Input: part model. Units: mm. Frame: model coordinates. Face numbers are marked on the shaded views. A direction names the side the tool comes from. Coordinates: 2 decimals unless noted, no trailing zeros. One line per question, with ' | ' between items. Start each with the question number.
```python
from build123d import *

# Parameters (mm, degrees)
F0_W     = 60
F0_H     = 52.3357634497
F0_R     = 16.5
F1_DEPTH = 11.80754
F3_DEPTH = 7.76524
F3_TAPER = -4
F4_R     = 5
F5_R     = 5


with BuildPart() as f1:
    # F0 (on Top) → F1 (new body)
    with BuildSketch(Plane.XY):
        Polygon((0, 78.3958006123), (-30, 26.1678817249), (30, 26.1678817249), align=None)
        Rectangle(F0_W, F0_H)
        Circle(F0_R, mode=Mode.SUBTRACT)
        Polygon((-30, -26.1678817249), (-30, 26.1678817249), (-72.2627720197, 0), align=None)
        Polygon((71.6058312025, 0), (30, 26.1678817249), (30, -26.1678817249), align=None)
        Polygon((30, -26.1678817249), (-30, -26.1678817249), (0, -77.8738003652), align=None)
    extrude(amount=-F1_DEPTH)

    # F2 (on Top) → F3 (join)
    with BuildSketch(Plane.XY):
        Polygon((56.5895004995, -64.7582306214), (0, 0), (-56.5895004995, -64.7582306214), align=None)
        Polygon((-56.5895004995, 64.7582306214), (0, 0), (56.5895004995, 64.7582306214), align=None)
    extrude(amount=-F3_DEPTH, taper=F3_TAPER)

    # F4
    f4_edges = [f1.edges().sort_by_distance(p)[0] for p in [
        (-57.187308, 65.02973, -3.88262),
        (-72.262772, 0, -5.90377),
        (-57.187308, -65.02973, -3.88262),
    ]]
    fillet(f4_edges, radius=F4_R)

    # F5
    f5_edges = [f1.edges().sort_by_distance(p)[0] for p in [
        (57.187308, 65.02973, -3.88262),
        (71.605831, 0, -5.90377),
        (57.187308, -65.02973, -3.88262),
    ]]
    fillet(f5_edges, radius=F5_R)


solid = f1.part
```
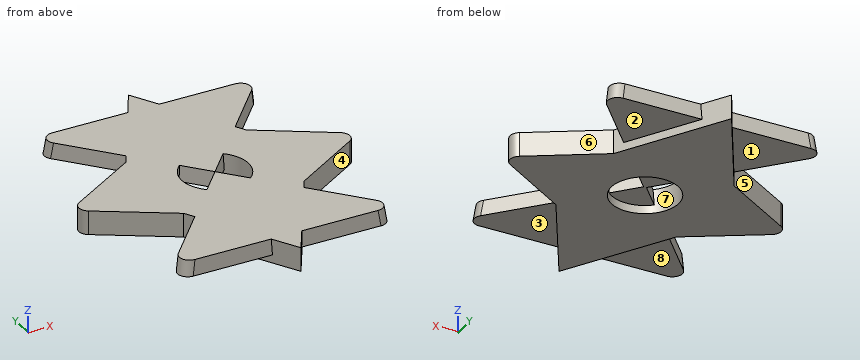
1) First-contact query: P1, Ø7, axis at x = -4, y = -5, coming from the -Z side; P2, Ø4, axis at x = -23, z = -10, coming from the -Y side; P3, Ø5, axis at y = 27, z = -7, coming from the +X side. Flat tips, straight axial feed; report the tip coordinate or a pass-through.
2) Pull-direction query (X, two-part tool) for the marked faces 6, 7 and 8; classes: released by +X, released by -X, zero draft, split by the parting line, or undercut.
3) Section A-A, the plane x = -39. Give the number of separate pieces and of enclosed holes in the cut face, then the cut area to 3 significant figures.
4) Ray query, line 1 (Y direction, x = -37, z = -4.75); line 2 (Y direction, x = 0, z = -8.75); line 3 (X direction, y = 11, z = -4.5). Return the intervals inside material, ascending.
5) Access query for the marked faces 1, 2, 3, 4 and 5. Directions: +Z, -Z, +X, -X, +Y, -Y. A direction counts if a zero-diameter tool reaches every point of the face in a straight line with its end or side. Return the directions, or none.
Answer block:
1) P1: stops at z = -7.77 | P2: stops at y = -41.68 | P3: stops at x = 32.65
2) face 6: released by +X | face 7: undercut | face 8: zero draft
3) separate pieces: 3 | enclosed holes: 0 | area: 810 mm2
4) line 1: y = -65.09 to -41.84, -21.83 to 21.83, 41.84 to 65.09 | line 2: y = -77.87 to -16.5, 16.5 to 78.4 | line 3: x = -54.5 to -12.3, -10.03 to 10.03, 12.3 to 54.12
5) face 1: -Z, -X, +Y | face 2: -Z, +X, +Y | face 3: -Z, +X, -Y | face 4: +Z, -Z, +X | face 5: +Z, -Z, -X
